Check sheet for the drawn part. Datum: minimum x, y, z corner. Units: mm. A direction names the side the tool comes from. Round coordinates to 2 decimals unless told otherwise and drop trailing zeros. Order: outer loops, then holes, each group sorted by start corner. A loop starts at its lowest first (then second) coordinate and runs counter-clockwise, first axis right, second up. Notation, with made-up numbers: (-33.75, 43.5) -> (1.25, 43.5) arc R21 ccw to (1.25, 58.5) -> close; hole circle Ø8 at (-2.5, 24.25). An arc over 180 degrees is marked (long way). Answer in a Markdown table with one row per item.
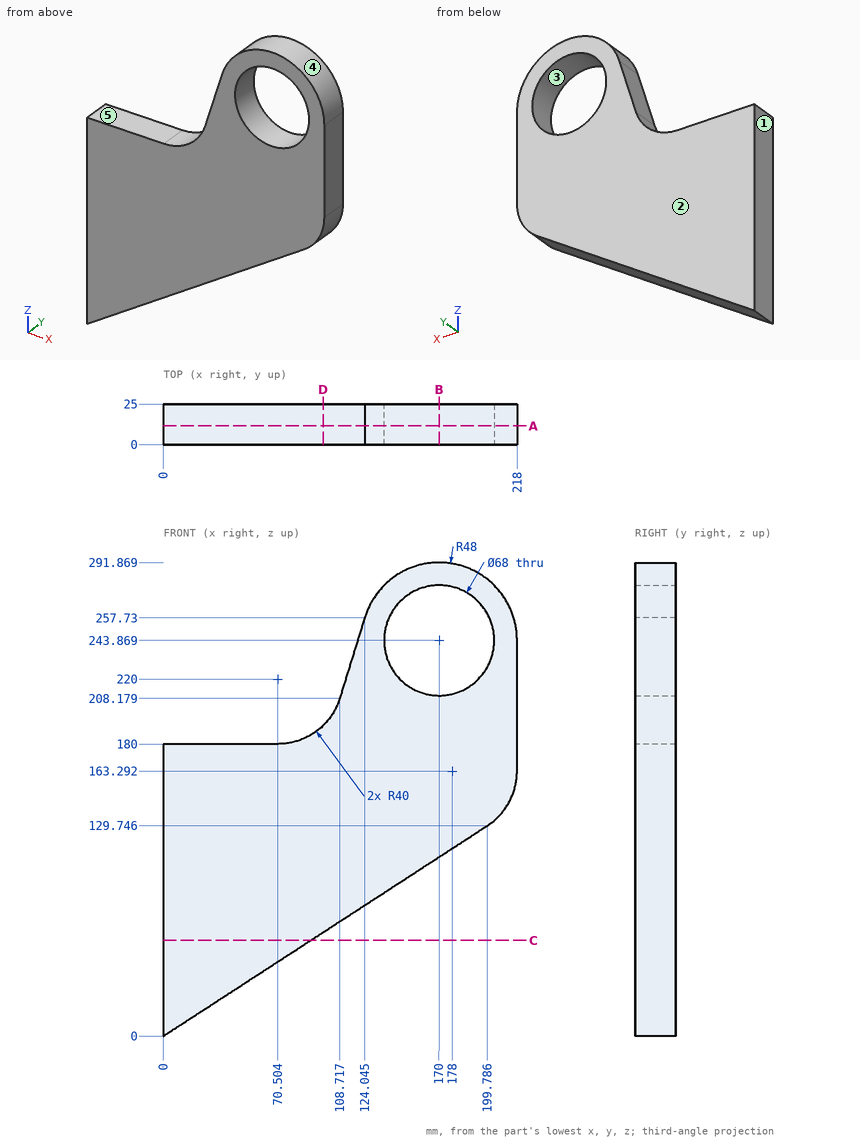
(1) Section check B-B on x = 170. Record the boundary of the cut face in (y, z).
Solutions:
| item | result |
|---|---|
| outline | (0, 110.4) -> (25, 110.4) -> (25, 209.87) -> (0, 209.87) -> close; (0, 277.87) -> (25, 277.87) -> (25, 291.87) -> (0, 291.87) -> close |
(2) Depth check by flat-ended pin: pin 1 Ø1 at (x, y) = (131.5, 8) entering from -Z (1 decimal); pin 2 Ø6 at (x, y) = (189.5, 17.5) entering from +Z; pin 3 Ø4 at (y, z) = (8, 261.5) entering from +X. Enter the tip coordinate at first touch or a pass-through.
Solutions:
| item | result |
|---|---|
| pin 1 | z = 85.1 |
| pin 2 | z = 288.94 |
| pin 3 | x = 215.38 |
(3) Scan lines: probe 1 along Z at (x, y) = (170, 15.75); probe 2 along Z at (x, y) = (175, 6.75); probe 3 along X at (y, z) = (4.5, 50) (1 decimal). Record each from-to range of solid material in increasing order. Write a range as from..to.
Solutions:
| item | result |
|---|---|
| probe 1 | 110.4..209.87, 277.87..291.87 |
| probe 2 | 113.65..210.24, 277.5..291.61 |
| probe 3 | 0..77 |
(4) Section check D-D on x = 98.5. Record the boundary of the cut face in (y, z), plus the area to 3 significant figures.
Solutions:
| item | result |
|---|---|
| outline | (0, 63.97) -> (25, 63.97) -> (25, 191.43) -> (0, 191.43) -> close |
| area | 3,190 mm^2 |
(5) Section check A-A on y = 11.5. Record the boundary of the cut face in (x, z) (1 decimal).
Solutions:
| item | result |
|---|---|
| outline | (0, 0) -> (199.8, 129.7) arc R40 ccw to (218, 163.3) -> (218, 243.9) arc R48 ccw to (124, 257.7) -> (108.7, 208.2) arc R40 cw to (70.5, 180) -> (0, 180) -> close; hole circle Ø68 at (170, 243.9) |
(6) Draft check along X on the marked faces 1, 2 and 3. Enter one of: pulls with the +X half, pulls with the -X half, needs draft (parallel to the pull), parting line crosses it, or undercut.
Solutions:
| item | result |
|---|---|
| face 1 | pulls with the -X half |
| face 2 | needs draft |
| face 3 | undercut |
(7) Tool access check on the marked faces 4 and 5. Record the directions out of +Z, -Z, +X, -X, +Y, -Y that give a thin tool (end or side, any length) a straight path to the whole face; none if there is none.
Solutions:
| item | result |
|---|---|
| face 4 | +Z, +Y, -Y |
| face 5 | +Z, -X, +Y, -Y |
(8) Section check C-C on z = 59. Record the boundary of the cut face in (x, y), plus the area to 3 significant figures.
Solutions:
| item | result |
|---|---|
| outline | (0, 0) -> (90.85, 0) -> (90.85, 25) -> (0, 25) -> close |
| area | 2,270 mm^2 |
